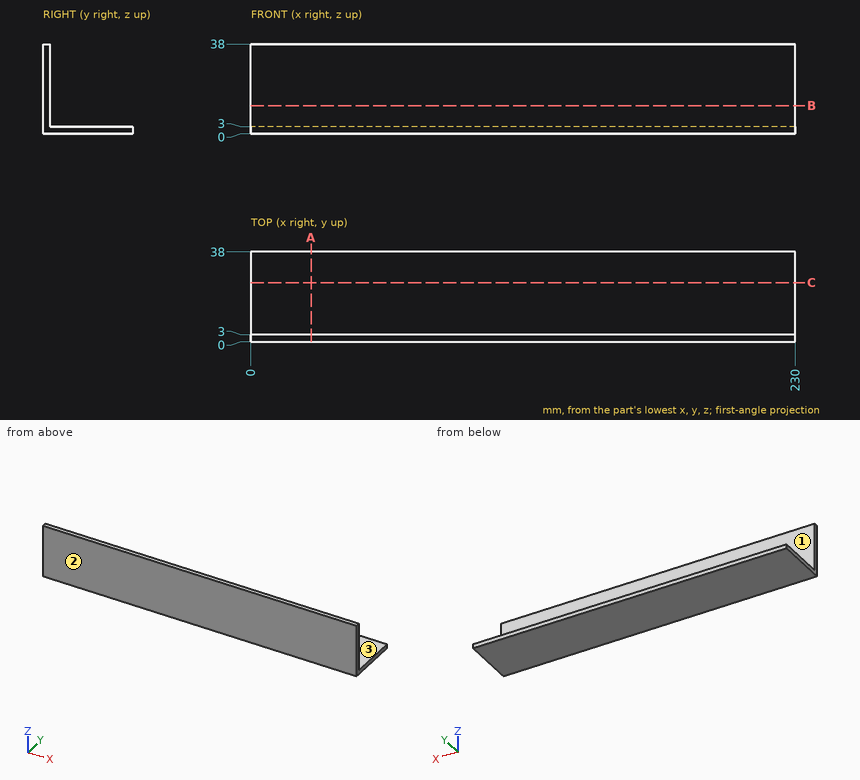
Geometry check sheet. Reference: drawing and pictorial views, mm from the part's lowest x, y, z. Coordinates: 2 decimals unless noted, no trailing zeros. Order: outer loops, then holes, each group sorted by start corner. A loop starts at its lowest first (then second) coordinate and runs counter-clockwise, first axis right, second up. Notation, with made-up numbers: M 37,-20 L 78,-20 A20 ccw 78,0 Z; hole C 81,83 d5. An arc over 180 degrees is marked long. Write each question's results on one line, items separated by ' | '. Start each with the question number.
1. Material ranges on probe 1 along Z at (x, y) = (172.5, 3.5), recorded low to high.
2. Mould release check, pull along Y, two halves, no side actions. Record for the marked faces 1, 2 and 3: +Y half, -Y half, draft (parallel to the pull), parting line (faces both ways), or undercut.
3. Cross-section at B-B on z = 12. Record the cut outline in (x, y).
4. Cross-section at A-A on x = 25.5. Record the cut outline in (y, z).
5. Go/stop test with flat-tipped pins: P1, Ø1, axis at x = 61, z = 22.5, coming from the -Y side; P2, Ø4, axis at x = 178, y = 20, coming from the +Z side; P3, Ø10.5, axis at x = 98, z = 28.5, coming from the +Y side. Record where each tip stops, or that it passes through.
Checks:
1) probe 1: z = 0 to 3
2) face 1: +Y half | face 2: -Y half | face 3: draft
3) outline: M 0,0 L 230,0 L 230,3 L 0,3 Z
4) outline: M 0,0 L 38,0 L 38,3 L 3,3 L 3,38 L 0,38 Z
5) P1: stops at y = 0 | P2: stops at z = 3 | P3: stops at y = 3
